```python
from build123d import *

# Parameters (mm, degrees)
CROQUIS1_R              = 5
SALIENTE_EXTRUIR1_DEPTH = 8
CROQUIS4_R              = 2.55
CORTAR_EXTRUIR1_DEPTH   = 4


with BuildPart() as part:
    # Croquis1 → Saliente-Extruir1 (new body)
    with BuildSketch(Plane.XY):
        Circle(CROQUIS1_R)
    extrude(amount=SALIENTE_EXTRUIR1_DEPTH)

    # Croquis3 → Cortar-Revolución2 (revolve, cut)
    with BuildSketch(Plane(origin=(0, 0, 0), x_dir=(0, 0, -1), z_dir=(1, 0, 0)), mode=Mode.PRIVATE) as cortar_revoluci_n2_sk:
        Polygon((-8, 3.970963049), (0, 5), (-8, 5), align=None)
    revolve(cortar_revoluci_n2_sk.sketch.rotate(Axis((0, 0, 8), (0, 0, -1)), 90), axis=Axis((0, 0, 8), (0, 0, -1)), mode=Mode.SUBTRACT)

    # Croquis4 → Cortar-Extruir1 (cut)
    with BuildSketch(Plane(origin=(0, 0, 0), x_dir=(-1, 0, 0), z_dir=(0, 0, -1))):
        Circle(CROQUIS4_R)
    extrude(amount=-CORTAR_EXTRUIR1_DEPTH, mode=Mode.SUBTRACT)


solid = part.part
```
Geometry check sheet. Reference: the model listing, model coordinates, mm. A direction names the side the tool comes from. Coordinates: 2 decimals unless noted, no trailing zeros. Write each loop counter-clockwise with the first axis right and the second up, starting at its lowest first coordinate (ties: lowest second). Pieces come first, ordered by that corner, then holes. Notation, with made-up numbers: M -6.5,31.25 L -1.5,31.25 A7 ccw -1.5,41.25 Z; hole C 56.5,89 d3. An arc over 180 degrees is marked long. Answer as a JSON object with one key per item and string values.
1. Section check C-C, the plane z = 2.75. Enter the section's corners in (x, y), plus the area to 3 significant figures.
Answers below:
{"outline": "C 0,0 d9.29; hole C 0,0 d5.1", "area": "47.4 mm²"}
2. Scan lines: L1, parallel to Y at x = -0.5, z = 3; L2, parallel to Z at x = -2, y = -1.5; L3, parallel to Y at x = 0.25, z = 2. Record each from-to range of solid material in increasing order.
Answers below:
{"L1": "y = -4.59 to -2.5, 2.5 to 4.59", "L2": "z = 4 to 8", "L3": "y = -4.74 to -2.54, 2.54 to 4.74"}
3. Section check A-A, the plane y = 0. Enter the section's corners in (x, z).
Answers below:
{"outline": "M -5,0 L -2.55,0 L -2.55,4 L 2.55,4 L 2.55,0 L 5,0 L 3.97,8 L -3.97,8 Z"}
4. Tool access check on faces 1 (the flat face through (0, 0, 4)), 2 (the flat face through (0, 0, 8)). Record the directions out of +Z, -Z, +X, -X, +Y, -Y that give a thin tool (end or side, any length) a straight path to the whole face; none if there is none.
Answers below:
{"face 1": "-Z", "face 2": "+Z, +X, -X, +Y, -Y"}
5. Go/stop test with flat-tipped pins: pin 1 Ø1.5 at (x, z) = (0.5, 4) entering from +Y; pin 2 Ø1 at (x, z) = (0, 1.5) entering from +Y; pin 3 Ø4 at (y, z) = (-2, 4.5) entering from +X. Record where each tip stops, or that it passes through.
Answers below:
{"pin 1": "stops at y = 4.57", "pin 2": "stops at y = 4.87", "pin 3": "stops at x = 4.57"}
6. Section check D-D, the plane z = 4.5. Enter the section's corners in (x, y), plus the area to 3 significant figures.
Answers below:
{"outline": "C 0,0 d8.84", "area": "61.4 mm²"}
